Autodesk Inventor part; units mm, degrees
ref_plane "YZ Plane" through (0, 0, 0) normal (1, 0, 0) x (0, 1, 0)
ref_plane "XZ Plane" through (0, 0, 0) normal (0, 1, 0) x (-1, 0, 0)
ref_plane "XY Plane" through (0, 0, 0) normal (0, 0, 1) x (1, 0, 0)
sketch "草图1" plane through (0, 0, 0) normal (0, 0, 1) x (1, 0, 0)
  line L0 (10, -10) -> (-10, -10)
  line L1 (-10, -10) -> (-10, 10)
  line L2 (-10, 10) -> (10, 10)
  line L3 (10, 10) -> (10, -10)
  line L4 (10, -10) -> (-10, 10) construction
  line L5 (-10, -10) -> (10, 10) construction
  point P0 (0, 0)
  dimension "d0" = 20
  dimension "d1" = 20
extrude "拉伸1" add sketch "草图1" along normal blind 100
sketch "草图2" plane through (0, 0, 100) normal (0, 0, 1) x (1, 0, 0)
  line L0 (-10.3453, 3.6494) -> (-10.3453, 10.3451)
  line L1 (-10.3453, 3.0994) -> (-10.3453, 10.3451)
  line L2 (-10.3453, 10.3451) -> (-10.3453, -10.0013)
  line L3 (-10.3453, 5.4994) -> (-10.3453, 10.3451)
  line L4 (-3.6495, 9.6435) -> (-3.0995, 9.6435)
  line L5 (-5.4995, 12.01) -> (-5.4995, 5.4994)
  line L6 (-3.0995, 10.3451) -> (-3.0995, 9.4451)
  line L7 (-5.4995, 9.4451) -> (0.0005, 9.4451)
  line L8 (-3.6495, 10.3451) -> (-3.6495, 9.4451)
  circle A0 centre (0.0005, -0.0006) radius 2.55
  line L9 (-5.4995, 10.3451) -> (-5.4995, 5.4994)
  line L10 (-10.3453, 10.3451) -> (-5.4995, 10.3451)
  line L11 (-5.4995, 5.4994) -> (-10.3453, 5.4994)
  line L12 (-4.2453, 4.2451) -> (-4.2453, -0.0006)
  line L13 (-10.3453, 10.3451) -> (-3.6495, 10.3451)
  line L14 (-10.3453, 10.3451) -> (-3.0995, 10.3451)
  line L15 (-11.061, -0.0006) -> (0.0005, -0.0006)
  line L16 (-1.0602, -0.0006) -> (-10.3453, 9.2845)
  line L17 (-10.3453, 10.3451) -> (0.0005, -0.0006)
  line L18 (0.0005, 1.06) -> (-9.2846, 10.3451)
  line L19 (0.0005, -0.0006) -> (0.0005, 11.5494)
  line L20 (10.0005, 10.3451) -> (-10.3453, 10.3451)
  line L21 (0.0005, 4.2451) -> (-4.2453, 4.2451)
  point P0 (0, 0)
  point P1 (-3.0995, 9.8951)
  point P2 (-5.4995, 6.56)
  point P3 (-3.1846, 4.2451)
  point P4 (0.0005, 10.3451)
  point P5 (-3.0995, 10.3451)
  dimension "d4" = 5.1
  dimension "d5" = 6.1
  dimension "d6" = 1.5
  dimension "d7" = 5.5
  dimension "d8" = 0.9
  dimension "d9" = 3.1
  dimension "d10" = 3.65
extrude "拉伸2" cut sketch "草图2" against normal blind 205.75 contours L5 L7 L19 L21 L18 | L16 L15 A0 | A0 L17 L15 L16 | L15 L19 A0 | A0 L18 L19 L17 | L14 L6 L4 L8 | A0 L19 L18 | L20 L19 L7 L6
mirror "镜像1" about plane through (0.0005, 10.3451, 100) normal (-1, 0, 0) of "拉伸2"
pattern_circular "环形阵列1" count 4 over 360 about axis through (0.0005, -0.0006, 100) along (0, 0, -1) of "拉伸2", "镜像1"
properties part number "铝方管2020x60"
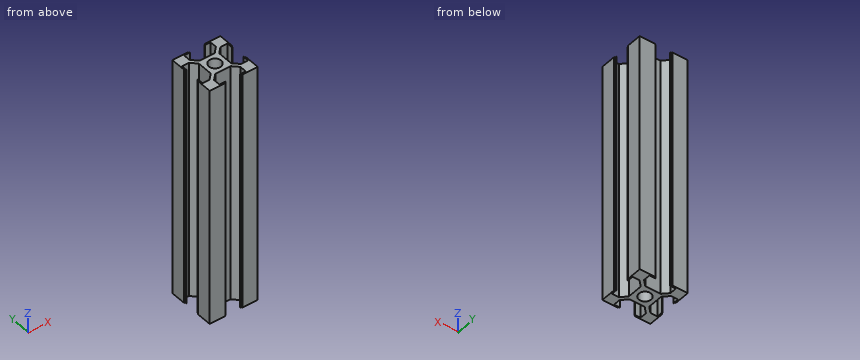
Can you work these out from the model? Positions are in its coordinate system, mm. Give positions to 0.01 mm unless a question says otherwise; leave off trailing zeros. Loops run counter-clockwise (first coordinate to the right, second up) from the corner with the lowest first, then second, coordinate; pieces in that order, holes last. Notation, with made-up numbers: M -28.5,6 L -17.5,6 A30 ccw -17.5,30 Z; hole C -37.5,54.5 d11. An arc over 180 degrees is marked long. One line per question, with ' | ' between items. Start each with the question number.
Q1. If we section it at A-A (y = 8.5): Please give me the cut outline in (x, z).
Q2. If I drill on line 1 (X direction, y = -7, z = 74.5); line 2 (X direction, y = 3.75, z = 33); line 3 (Y direction, x = 3.25, z = 87.5), over which ranges is the centre line in solid material (lowest first)? Write a range as from..to.
Q3. For pin 1 Ø3 at (x, z) = (-1.5, 73) entering from +Y, with a flat end and sliding along its axis, tell me the tip position at first contact or that it passes through.
Computed:
1) outline: M -10,0 L -5.5,0 L -5.5,100 L -10,100 Z; M 5.5,0 L 10,0 L 10,100 L 5.5,100 Z
2) line 1: x = -10..-5.5, 5.5..10 | line 2: x = -10..-9.45, -4.81..4.81, 9.45..10 | line 3: y = -9.64..-9.45, -4.31..4.31, 9.45..9.64
3) pin 1: stops at y = 4.25
